Autodesk Inventor part; units mm, degrees
ref_plane "Work Plane1" through (-145.9923, 42.0074, 2.54) normal (-1, 0, 0) x (0, 0, 1)
ref_plane "Work Plane2" through (-172.0273, 55.2154, 2.54) normal (0, -1, 0) x (1, 0, 0)
ref_plane "YZ Plane" through (0, 0, 0) normal (1, 0, 0) x (0, 1, 0)
sketch "Sketch1" plane through (0, 0, 0) normal (0, 0, 1) x (1, 0, 0)
  line L0 (-172.0273, 68.4234) -> (-119.9573, 68.4234)
  line L1 (-119.9573, 68.4234) -> (-119.9573, 42.0074)
  line L2 (-119.9573, 42.0074) -> (-172.0273, 42.0074)
  line L3 (-172.0273, 42.0074) -> (-172.0273, 68.4234)
  point P0 (0, 0)
  dimension "d0" = 52.07
  dimension "d1" = 26.416
extrude "Extrusion1" add sketch "Sketch1" along normal blind 2.54
sketch "Sketch2" plane through (0, 0, 2.54) normal (0, 0, 1) x (1, 0, 0)
  line L0 (-119.9573, 68.4234) -> (-172.0273, 68.4234)
  line L1 (-119.9573, 68.4234) -> (-172.0273, 68.4234)
  line L2 (-172.0273, 68.4234) -> (-172.0273, 42.0074)
  line L3 (-172.0273, 42.0074) -> (-119.9573, 42.0074)
  line L4 (-119.9573, 42.0074) -> (-119.9573, 68.4234)
  line L5 (-116.7823, 38.8324) -> (-175.2023, 38.8324)
  line L6 (-175.2023, 38.8324) -> (-175.2023, 71.5984)
  line L7 (-175.2023, 71.5984) -> (-116.7823, 71.5984)
  line L8 (-116.7823, 71.5984) -> (-116.7823, 38.8324)
  point P0 (0, 0)
  dimension "d18" = 3.175
  dimension "d19" = 3.175
  dimension "d20" = 3.175
  dimension "d21" = 3.175
  dimension "d25" = 32.766
  dimension "d26" = 58.42
extrude "Extrusion2" add sketch "Sketch2" along normal blind 2.54 contours L4 L3 L2 L0 | L5 L6 L7 L8
fillet "Fillet1" radius 3.175 4 edges at (-116.7823, 38.8324, 3.81) (-175.2023, 38.8324, 3.81) (-116.7823, 71.5984, 3.81) (-175.2023, 71.5984, 3.81)
sketch "Sketch4" plane through (0, 0, 5.08) normal (0, 0, 1) x (1, 0, 0)
  circle A0 centre (-175.5648, 71.9609) radius 1.3891
  line L0 (-119.9573, 71.5984) -> (-172.0273, 71.5984)
  arc A1 (-172.0273, 71.5984) -> (-175.2023, 68.4234) centre (-172.0273, 68.4234) ccw
  line L1 (-175.2023, 68.4234) -> (-175.2023, 42.0074)
  arc A2 (-172.0273, 71.5984) -> (-175.2023, 68.4234) centre (-175.5648, 71.9609) ccw
  point P0 (0, 0)
  dimension "d12" = 2.7781
  dimension "d23" = 3.556
extrude "Extrusion3" add sketch "Sketch4" against normal up to surface (2.54 mm away)
ref_plane "Work Plane1" through (-145.9923, 42.0074, 2.54) normal (-1, 0, 0) x (0, 0, 1)
ref_plane "Work Plane2" through (-172.0273, 55.2154, 2.54) normal (0, -1, 0) x (1, 0, 0)
mirror "Mirror1" about plane through (-145.9923, 42.0074, 2.54) normal (-1, 0, 0) of "Extrusion3"
mirror "Mirror2" about plane through (-172.0273, 55.2154, 2.54) normal (0, -1, 0) of "Extrusion3", "Mirror1"
fillet "Fillet3" radius 3.175 8 edges at (-175.2023, 42.0074, 3.81) (-175.2023, 68.4234, 3.81) (-119.9573, 38.8324, 3.81) (-172.0273, 71.5984, 3.81) (-119.9573, 71.5984, 3.81) (-116.7823, 68.4234, 3.81) (-116.7823, 42.0074, 3.81) (-172.0273, 38.8324, 3.81)
equation "\"d19\" = d18"
equation "\"d21\" = d20"
properties part number "sensor_lid"
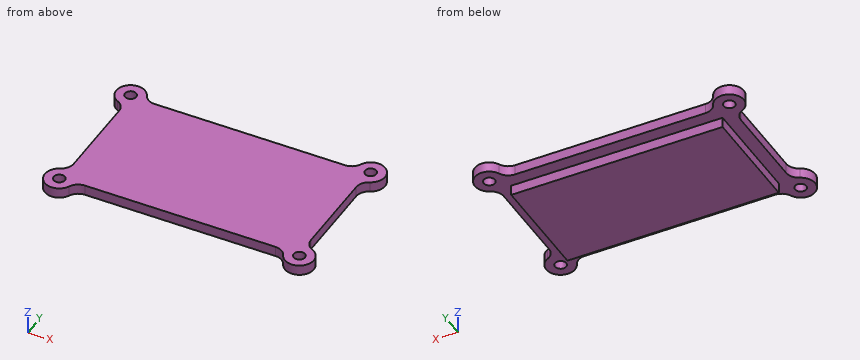
Build history of the part. All positions in model axes, mm. Round coordinates to 2 decimals unless told otherwise and drop trailing zeros. Loops run counter-clockwise (first coordinate to the right, second up) from the corner with the lowest first, then second, coordinate; pieces in that order, holes last. Notation, with made-up numbers: (77.5, 14.5) -> (94.5, 14.5) arc R16 cw to (94.5, 36.5) -> close; hole circle Ø2 at (53.5, 34.5). An arc over 180 degrees is marked (long way). Answer in a Markdown table with one row per item.
Item 1: Pin check, flat tips, straight feed: pin 1 (0.8 mm diameter, centred on y = 54.5, z = 3.5, fed in from -X); pin 2 (0.8 mm diameter, centred on y = 51, z = 4.5, fed in from +X); pin 3 (4.5 mm diameter, centred on x = -175.56, y = 38.47, fed in from -Z); pin 4 (3 mm diameter, centred on x = -168, y = 53.5, fed in from -Z). Stop position of each tip, or through.
Answers below:
| item | result |
|---|---|
| pin 1 | stops at x = -175.2 |
| pin 2 | stops at x = -116.78 |
| pin 3 | stops at z = 2.54 |
| pin 4 | stops at z = 0 |
Item 2: Drill centre lines: L1, parallel to X at y = 57.5, z = 4.05; L2, parallel to Y at x = -143, z = 1.15; L3, parallel to Y at x = -138, z = 3.4. Where is each one in solid material? Low to high. Write a range as [from, to].
Answers below:
| item | result |
|---|---|
| L1 | x = [-175.2, -116.78] |
| L2 | y = [42.01, 68.42] |
| L3 | y = [38.83, 71.6] |
Item 3: Saw through at B-B (y = 57.5). Write the cut outline in (x, z).
Answers below:
| item | result |
|---|---|
| outline | (-175.2, 2.54) -> (-172.03, 2.54) -> (-172.03, 0) -> (-119.96, 0) -> (-119.96, 2.54) -> (-116.78, 2.54) -> (-116.78, 5.08) -> (-175.2, 5.08) -> close |
Item 4: Saw through at A-A (x = -124.5). Write the cut outline in (y, z), and give its area (3 significant figures).
Answers below:
| item | result |
|---|---|
| outline | (38.83, 2.54) -> (42.01, 2.54) -> (42.01, 0) -> (68.42, 0) -> (68.42, 2.54) -> (71.6, 2.54) -> (71.6, 5.08) -> (38.83, 5.08) -> close |
| area | 150 mm² |
Item 5: Saw through at C-C (z = 3.4). Write the cut outline in (x, y) (3 decimals).
Answers below:
| item | result |
|---|---|
| outline | (-177.051, 41.701) arc R3.556 ccw (long way) to (-172.334, 36.984) arc R3.175 cw to (-169.45, 38.832) -> (-122.535, 38.832) arc R3.175 cw to (-119.651, 36.984) arc R3.556 ccw (long way) to (-114.934, 41.701) arc R3.175 cw to (-116.782, 44.585) -> (-116.782, 65.846) arc R3.175 cw to (-114.934, 68.73) arc R3.556 ccw (long way) to (-119.651, 73.447) arc R3.175 cw to (-122.535, 71.598) -> (-169.45, 71.598) arc R3.175 cw to (-172.334, 73.447) arc R3.556 ccw (long way) to (-177.051, 68.73) arc R3.175 cw to (-175.202, 65.846) -> (-175.202, 44.585) arc R3.175 cw to start; hole circle Ø2.778 at (-175.565, 38.47); hole circle Ø2.778 at (-175.565, 71.961); hole circle Ø2.778 at (-116.42, 38.47); hole circle Ø2.778 at (-116.42, 71.961) |
